Verification items for the finished model (mm, model axes). A direction names the side the tool comes from. Give positions to 0.01 mm unless a question says otherwise; leave off trailing zeros. Order: outer loops, then holes, each group sorted by start corner. A loop starts at its lowest first (then second) coordinate and runs counter-clockwise, first axis right, second up. Notation, with made-up numbers: (89, 47) -> (117, 47) arc R15 cw to (117, 65) -> close; hole circle Ø7 at (-25.75, 20.5). An arc over 180 degrees is marked (long way). Return JSON: item names as keys, results as strings. Group by question number.
(1) Depth check by flat-ended pin: pin 1 Ø2 at (y, z) = (-4.5, -8.5) entering from -X; pin 2 Ø12 at (y, z) = (-8, 1.5) entering from +X. Enter the tip coordinate at first touch or a pass-through.
(2) Tool access check on faces 4 (the face through (-1, -12.7, 0)), 5 (the face through (-1, 0, -11.049)). Record the directions out of +Z, -Z, +X, -X, +Y, -Y that give a thin tool (end or side, any length) a straight path to the whole face; none if there is none.
(3) Cross-section at A-A on z = -3.5. Enter the section's corners in (x, y), then the cut area to 3 significant figures.
(4) Thickness scan on line 1 along Y through (x, z) = (-57, -8); line 2 along Y through (x, z) = (31, -10.5). Record the ranges inside material, lowest first.
(5) Release check for a two-part mould opening along Z. For faces 1 (the face through (-4, 11.049, 0)), 2 (the face through (-4, 12.7, 0)), 3 (the face through (-1, 0, -12.7)) record: pulls with the +Z half, pulls with the -Z half, needs draft (parallel to the pull), parting line crosses it, or undercut.
(6) Cross-section at C-C on x = 28. Enter the section's corners in (y, z).
(7) Cross-section at B-B on y = -7. Enter the section's corners in (x, z), then the cut area to 3 significant figures.
from build123d import *

# Parameters (mm, degrees)
BOSS_EXTRUDE1_DEPTH      = 76.2
BOSS_EXTRUDE1_DEPTH_BACK = 76.2
CUT_EXTRUDE1_DEPTH       = 82.319677815


with BuildPart() as part:
    # Sketch4 → Boss-Extrude1 (new, two sides: drawn at the far end of the back side and taken through both)
    with BuildSketch(Plane(origin=(0, 0, 0), x_dir=(0, 0, -1), z_dir=(1, 0, 0)).offset(-BOSS_EXTRUDE1_DEPTH_BACK)):
        with BuildLine():
            Line((12.7, -11.43), (12.7, 11.43))
            ThreePointArc((12.7, 11.43), (12.328025612, 12.328025612), (11.43, 12.7))
            Line((11.43, 12.7), (-11.43, 12.7))
            ThreePointArc((-11.43, 12.7), (-12.328025612, 12.328025612), (-12.7, 11.43))
            Line((-12.7, 11.43), (-12.7, -11.43))
            ThreePointArc((-12.7, -11.43), (-12.328025612, -12.328025612), (-11.43, -12.7))
            Line((-11.43, -12.7), (11.43, -12.7))
            ThreePointArc((11.43, -12.7), (12.328025612, -12.328025612), (12.7, -11.43))
        make_face()
        with BuildLine():
            Line((11.049, 9.9441), (11.049, -9.9441))
            ThreePointArc((11.049, -9.9441), (10.725382283, -10.725382283), (9.9441, -11.049))
            Line((9.9441, -11.049), (-9.9441, -11.049))
            ThreePointArc((-9.9441, -11.049), (-10.725382283, -10.725382283), (-11.049, -9.9441))
            Line((-11.049, -9.9441), (-11.049, 9.9441))
            ThreePointArc((-11.049, 9.9441), (-10.725382283, 10.725382283), (-9.9441, 11.049))
            Line((-9.9441, 11.049), (9.9441, 11.049))
            ThreePointArc((9.9441, 11.049), (10.725382283, 10.725382283), (11.049, 9.9441))
        make_face(mode=Mode.SUBTRACT)
    extrude(amount=BOSS_EXTRUDE1_DEPTH + BOSS_EXTRUDE1_DEPTH_BACK)

    # Sketch5 → Cut-Extrude1 (cut, through all)
    with BuildSketch(Plane.XY.offset(12.7)):
        Polygon((76.2, -12.7), (70.568955569, 12.7), (76.2, 12.7), align=None)
    extrude(amount=-CUT_EXTRUDE1_DEPTH, mode=Mode.SUBTRACT)


solid = part.part
Verdict:
{
 "1": {"pin 1": "through", "pin 2": "x = 76.2"},
 "2": {"face 4": "+Z, -Z, +X, -X, -Y", "face 5": "+X, -X"},
 "3": {"outline": "(-76.2, -12.7) -> (76.2, -12.7) -> (75.83, -11.05) -> (-76.2, -11.05) -> close; (-76.2, 11.05) -> (70.93, 11.05) -> (70.57, 12.7) -> (-76.2, 12.7) -> close", "area": "494 mm²"},
 "4": {"line 1": "-12.7 to -11.05, 11.05 to 12.7", "line 2": "-12.7 to -10.9, 10.9 to 12.7"},
 "5": {"face 1": "undercut", "face 2": "needs draft", "face 3": "pulls with the -Z half"},
 "6": {"outline": "(-12.7, -11.43) arc R1.27 ccw to (-11.43, -12.7) -> (11.43, -12.7) arc R1.27 ccw to (12.7, -11.43) -> (12.7, 11.43) arc R1.27 ccw to (11.43, 12.7) -> (-11.43, 12.7) arc R1.27 ccw to (-12.7, 11.43) -> close; hole (-11.05, -9.94) arc R1.1 ccw to (-9.94, -11.05) -> (9.94, -11.05) arc R1.1 ccw to (11.05, -9.94) -> (11.05, 9.94) arc R1.1 ccw to (9.94, 11.05) -> (-9.94, 11.05) arc R1.1 ccw to (-11.05, 9.94) -> close"},
 "7": {"outline": "(-76.2, -12.7) -> (74.94, -12.7) -> (74.94, -11.05) -> (-76.2, -11.05) -> close; (-76.2, 11.05) -> (74.94, 11.05) -> (74.94, 12.7) -> (-76.2, 12.7) -> close", "area": "499 mm²"}
}
